Geometry: see drawing. Coordinates: mm, zero at the bounding-box minimum. A direction names the side the tool comes from. Round coordinates to 2 decimals unless told otherwise and drop trailing zeros. Write each loop counter-clockwise with the first axis right and the second up, starting at its lowest first coordinate (ties: lowest second). Pieces come first, ordered by that corner, then holes.
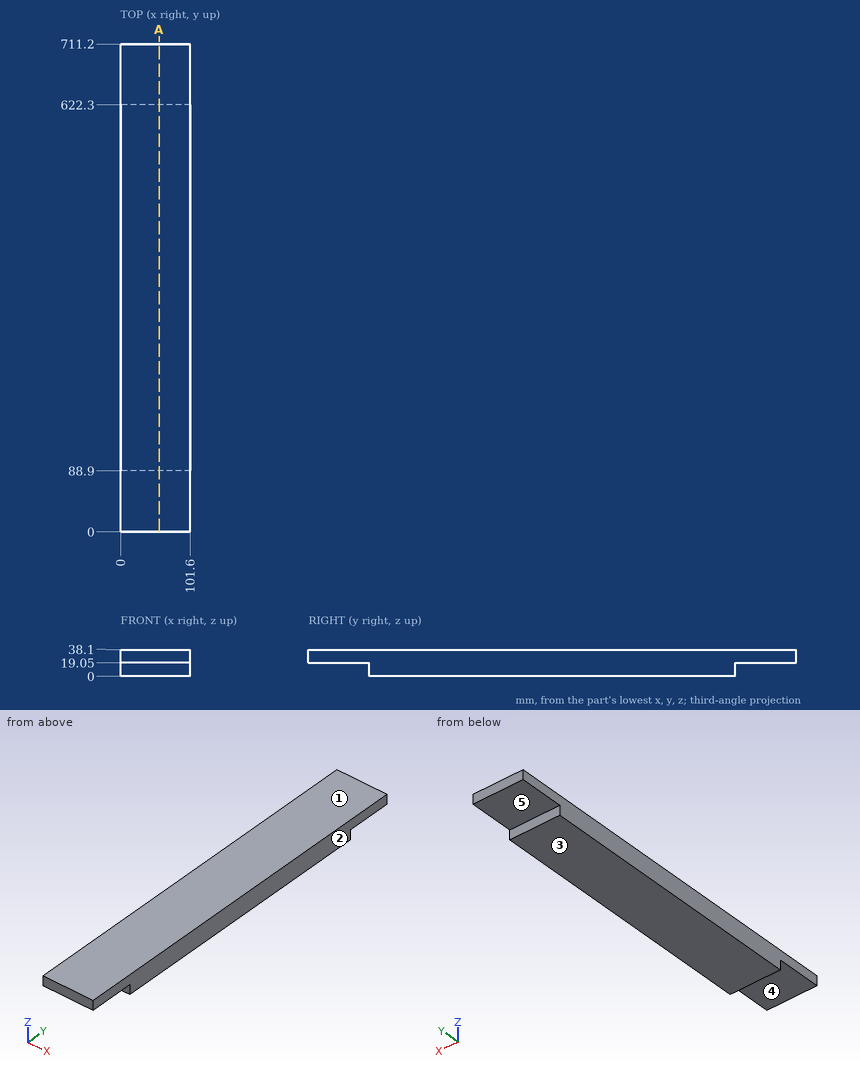
Q1. Set-up query: the marked faces 3, 4 and 5. Return all of +Z, -Z, +X, -X, +Y, -Y with unobstructed straight access to the full face (end or side cutting, diameter ignored); none if empty.
Q2. Mould query, pull axis X, two halves, no side actions, for the marked faces 1 and 2. Classes: pulls with the +X half, pulls with the -X half, needs draft (parallel to the pull), parting line crosses it, or undercut.
Q3. Pin query (flat end, axial travel): P1, Ø1, axis at x = 56.5, z = 6, coming from the +Y side; P2, Ø8, axis at x = 45.5, z = 7.5, coming from the -Y side. Return the tip coordinate at first contact, or that it passes through.
Q4. Section query A-A, the plane x = 56. Output: boundary loops of the cut face in (y, z), and give its area (3 significant figures).
Q5. Line query: line 1 (Z direction, x = 82.5, y = 36); line 2 (Y direction, x = 7, z = 3). Output: solid intervals per line, ascending.
Filled in:
1. face 3: -Z, +X, -X, +Y, -Y
1. face 4: -Z, +X, -X, -Y
1. face 5: -Z, +X, -X, +Y
2. face 1: needs draft
2. face 2: pulls with the +X half
3. P1: stops at y = 622.3
3. P2: stops at y = 88.9
4. outline: (0, 19.05) - (88.9, 19.05) - (88.9, 0) - (622.3, 0) - (622.3, 19.05) - (711.2, 19.05) - (711.2, 38.1) - (0, 38.1) - close
4. area: 23,700 mm2
5. line 1: z = 19.05 to 38.1
5. line 2: y = 88.9 to 622.3
